Source: CAD feature listing. Evaluate the final solid. Frame: model axes, mm. Face numbers are marked on the shaded views. A direction names the side the tool comes from. Give positions to 0.01 mm unless a question says otherwise; leave off trailing zeros. Write each loop counter-clockwise with the first axis right and the second up, starting at its lowest first coordinate (ties: lowest second). Pieces come first, ordered by that corner, then holes. Notation, with made-up numbers: M 34,60 L 76,60 A5 cw 76,64 Z; hole C 32.25,13 d4. An arc over 180 degrees is marked long. Return JSON: item names as keys, results as strings.
```python
from build123d import *

# Parameters (mm, degrees)
SKETCH_1_W          = 25
SKETCH_1_H          = 25
SKETCH_1_W_2        = 20.2
SKETCH_1_H_2        = 16.5
EXTRUDE_1_DEPTH     = 20
SKETCH_1_3_W        = 25
SKETCH_1_3_H        = 25
EXTRUDE_3_DEPTH     = 2
SKETCH_1_5_R        = 0.5
CUT_EXTRUDE_1_DEPTH = 0.1
SKETCH_2_R          = 0.95
CUT_EXTRUDE_2_DEPTH = 4
SKETCH_3_R          = 0.95
CUT_EXTRUDE_3_DEPTH = 4
CUT_EXTRUDE_START   = -4
SKETCH_4_R          = 0.95
CUT_EXTRUDE_4_DEPTH = 4
SKETCH_5_R          = 0.95
CUT_EXTRUDE_5_DEPTH = 4
SKETCH_6_R          = 0.75
CUT_EXTRUDE_6_DEPTH = 2


with BuildPart() as part:
    # 草图1 → 凸台-拉伸1 (new body)
    with BuildSketch(Plane(origin=(0, 0, 0), x_dir=(0, 0, -1), z_dir=(1, 0, 0))):
        Rectangle(SKETCH_1_W, SKETCH_1_H)
        Rectangle(SKETCH_1_W_2, SKETCH_1_H_2, mode=Mode.SUBTRACT)
    extrude(amount=EXTRUDE_1_DEPTH)

    # 草图1<3> → 凸台-拉伸3 (add)
    with BuildSketch(Plane(origin=(0, 0, 0), x_dir=(0, 0, -1), z_dir=(1, 0, 0))):
        Rectangle(SKETCH_1_3_W, SKETCH_1_3_H)
    extrude(amount=-EXTRUDE_3_DEPTH)

    # 草图1<5> → 切除-拉伸1 (cut)
    with BuildSketch(Plane(origin=(0, 0, 0), x_dir=(0, 0, -1), z_dir=(1, 0, 0))):
        Circle(SKETCH_1_5_R)
    extrude(amount=-CUT_EXTRUDE_1_DEPTH, mode=Mode.SUBTRACT)

    # 草图2 → 切除-拉伸2 (cut)
    with BuildSketch(Plane.XZ.offset(12.5)):
        with Locations(Location((2, 0, 0), (0, 0, 270))):
            Circle(SKETCH_2_R)
    extrude(amount=-CUT_EXTRUDE_2_DEPTH, mode=Mode.SUBTRACT)

    # 草图3 → 切除-拉伸3 (cut)
    with BuildSketch(Plane(origin=(0, 0, -12.5), x_dir=(-1, 0, 0), z_dir=(0, 0, -1))):
        with Locations((-2, 0)):
            Circle(SKETCH_3_R)
    extrude(amount=-CUT_EXTRUDE_3_DEPTH, mode=Mode.SUBTRACT)

    # 草图4 → 切除-拉伸4 (cut)
    with BuildSketch(Plane(origin=(0, 12.5, 0), x_dir=(1, 0, 0), z_dir=(0, 1, 0)).offset(CUT_EXTRUDE_START)):
        with Locations(Location((2, 0, 0), (0, 0, 90))):
            Circle(SKETCH_4_R)
    extrude(amount=CUT_EXTRUDE_4_DEPTH, mode=Mode.SUBTRACT)

    # 草图5 → 切除-拉伸5 (cut)
    with BuildSketch(Plane.XY.offset(12.5).offset(CUT_EXTRUDE_START)):
        with Locations(Location((2, 0, 0), (0, 0, 180))):
            Circle(SKETCH_5_R)
    extrude(amount=CUT_EXTRUDE_5_DEPTH, mode=Mode.SUBTRACT)

    # 草图6 → 切除-拉伸6 (cut)
    with BuildSketch(Plane.ZY.offset(2)):
        with Locations((-6.1, 0)):
            Circle(SKETCH_6_R)
        with Locations((6.1, 0)):
            Circle(SKETCH_6_R)
    extrude(amount=-CUT_EXTRUDE_6_DEPTH, mode=Mode.SUBTRACT)


solid = part.part
```
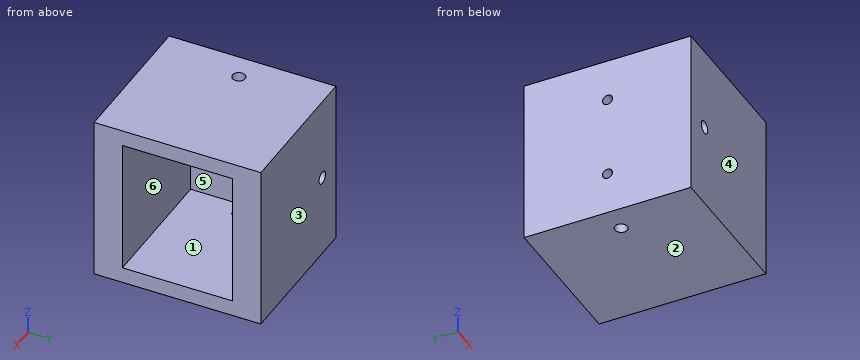
1) Contact query for flat-ended pins moving along their axis: pin 1 Ø1.2 at (y, z) = (0, 6.1) entering from +X; pin 2 Ø1.5 at (x, z) = (2, 0) entering from +Y; pin 3 Ø0.8 at (y, z) = (0, 0) entering from +X; pin 4 Ø6 at (y, z) = (5, 3) entering from +X. Output: stop coordinate, or through.
Numbers:
{"pin 1": "passes through", "pin 2": "stops at y = 8.5", "pin 3": "stops at x = -0.1", "pin 4": "stops at x = 0"}
2) Line query: line 1 (X direction, y = 10.6, z = 0); line 2 (Y direction, x = 3, z = 9.25); line 3 (Z direction, x = 7, y = -1). Output: solid intervals per line, ascending. Write a range as [from, to].
Numbers:
{"line 1": "x = [-2, 1.05], [2.95, 20]", "line 2": "y = [-12.5, -8.25], [8.25, 12.5]", "line 3": "z = [-12.5, -10.1], [10.1, 12.5]"}
3) Cut plane C-C, the plane x = 2. Return the cut outline in (y, z).
Numbers:
{"outline": "M -12.5,-12.5 L -0.95,-12.5 L -0.95,-10.1 L -8.25,-10.1 L -8.25,10.1 L -0.95,10.1 L -0.95,12.5 L -12.5,12.5 L -12.5,0.95 L -8.5,0.95 L -8.5,-0.95 L -12.5,-0.95 Z; M 0.95,-12.5 L 12.5,-12.5 L 12.5,-0.95 L 8.5,-0.95 L 8.5,0.95 L 12.5,0.95 L 12.5,12.5 L 0.95,12.5 L 0.95,10.1 L 8.25,10.1 L 8.25,-10.1 L 0.95,-10.1 Z"}
4) Set-up query: the marked faces 1 and 2. Return all of +Z, -Z, +X, -X, +Y, -Y with unobstructed straight access to the full face (end or side cutting, diameter ignored); none if empty.
Numbers:
{"face 1": "+X", "face 2": "-Z, +X, -X, +Y, -Y"}
5) Draft query along Y for the marked faces 3, 4, 5 and 6. Return one class per face: released by +Y, released by -Y, zero draft, split by the parting line, or undercut.
Numbers:
{"face 3": "released by +Y", "face 4": "released by -Y", "face 5": "undercut", "face 6": "undercut"}
6) Cut plane A-A, the plane z = 6.1. Return the cut outline in (x, y), then the cut area to 3 significant figures.
Numbers:
{"outline": "M -2,-12.5 L 20,-12.5 L 20,-8.25 L 0,-8.25 L 0,-0.75 L -2,-0.75 Z; M -2,0.75 L 0,0.75 L 0,8.25 L 20,8.25 L 20,12.5 L -2,12.5 Z", "area": "217 mm²"}
7) Cut plane B-B, the plane y = 0. Return the cut outline in (x, z).
Numbers:
{"outline": "M -2,-12.5 L 1.05,-12.5 L 1.05,-10.1 L 0,-10.1 L 0,-6.85 L -2,-6.85 Z; M -2,-5.35 L 0,-5.35 L 0,-0.5 L -0.1,-0.5 L -0.1,0.5 L 0,0.5 L 0,5.35 L -2,5.35 Z; M -2,6.85 L 0,6.85 L 0,10.1 L 1.05,10.1 L 1.05,12.5 L -2,12.5 Z; M 2.95,-12.5 L 20,-12.5 L 20,-10.1 L 2.95,-10.1 Z; M 2.95,10.1 L 20,10.1 L 20,12.5 L 2.95,12.5 Z"}
8) Cut plane D-D, the plane z = 0. Return the cut outline in (x, y).
Numbers:
{"outline": "M -2,-12.5 L 1.05,-12.5 L 1.05,-8.5 L 2.95,-8.5 L 2.95,-12.5 L 20,-12.5 L 20,-8.25 L 0,-8.25 L 0,-0.5 L -0.1,-0.5 L -0.1,0.5 L 0,0.5 L 0,8.25 L 20,8.25 L 20,12.5 L 2.95,12.5 L 2.95,8.5 L 1.05,8.5 L 1.05,12.5 L -2,12.5 Z"}
